from build123d import *

# Parameters (mm, degrees)
BOSS_EXTRUDE1_DEPTH = 4.5
SKETCH4_R           = 12.55
CUT_EXTRUDE1_DEPTH  = 2
CUT_EXTRUDE2_REACH  = 42.016
SKETCH5_R           = 2.1
SKETCH5_R_2         = 3.6
SKETCH8_W           = 3.5
SKETCH8_H           = 17
BOSS_EXTRUDE3_DEPTH = 20
FILLET3_R           = 10
FILLET4_R           = 10
SKETCH9_R           = 1.6
CUT_EXTRUDE3_DEPTH  = 68.190127898


with BuildPart() as part:
    # Sketch3 → Boss-Extrude1 (new body)
    with BuildSketch(Plane.XY):
        Polygon((-7.128665208, 13.142231947), (18.871334792, 13.142231947), (18.871334792, 2.142231947), (37.071334792, 2.142231947), (37.071334792, -14.857768053), (-25.328665208, -14.857768053), (-25.328665208, 2.142231947), (-7.128665208, 2.142231947), align=None)
    extrude(amount=BOSS_EXTRUDE1_DEPTH)

    # Sketch4 → Cut-Extrude1 (cut)
    with BuildSketch(Plane(origin=(0, 0, 0), x_dir=(-1, 0, 0), z_dir=(0, 0, -1))):
        with Locations((-5.871334792, 0.142231947)):
            Circle(SKETCH4_R)
    extrude(amount=-CUT_EXTRUDE1_DEPTH, mode=Mode.SUBTRACT)

    # Sketch5 → Cut-Extrude2 (cut, up to next)
    with BuildSketch(Plane(origin=(0, 0, 2), x_dir=(-1, 0, 0), z_dir=(0, 0, -1)), mode=Mode.PRIVATE) as cut_extrude2_sk1:
        with Locations((-14.621334792, 0.142231947)):
            Circle(SKETCH5_R)
    cut_extrude2_tool1 = extrude(cut_extrude2_sk1.sketch, amount=-CUT_EXTRUDE2_REACH, mode=Mode.PRIVATE) & part.part
    # Sketch5 → Cut-Extrude2 (cut, up to next)
    with BuildSketch(Plane(origin=(0, 0, 2), x_dir=(-1, 0, 0), z_dir=(0, 0, -1)), mode=Mode.PRIVATE) as cut_extrude2_sk2:
        with Locations(Location((2.878665208, 0.142231947, 0), (0, 0, 180))):
            Circle(SKETCH5_R)
    cut_extrude2_tool2 = extrude(cut_extrude2_sk2.sketch, amount=-CUT_EXTRUDE2_REACH, mode=Mode.PRIVATE) & part.part
    # Sketch5 → Cut-Extrude2 (cut, up to next)
    with BuildSketch(Plane(origin=(0, 0, 2), x_dir=(-1, 0, 0), z_dir=(0, 0, -1)), mode=Mode.PRIVATE) as cut_extrude2_sk3:
        with Locations((-5.871334792, 0.142231947)):
            Circle(SKETCH5_R_2)
    cut_extrude2_tool3 = extrude(cut_extrude2_sk3.sketch, amount=-CUT_EXTRUDE2_REACH, mode=Mode.PRIVATE) & part.part
    add(cut_extrude2_tool1.solids().sort_by_distance((14.621335, 0.142232, 2))[0], mode=Mode.SUBTRACT)
    add(cut_extrude2_tool2.solids().sort_by_distance((-2.878665, 0.142232, 2))[0], mode=Mode.SUBTRACT)
    add(cut_extrude2_tool3.solids().sort_by_distance((5.871335, 0.142232, 2))[0], mode=Mode.SUBTRACT)

    # Sketch8 → Boss-Extrude3 (add)
    with BuildSketch(Plane(origin=(0, 0, 0), x_dir=(-1, 0, 0), z_dir=(0, 0, -1))):
        with Locations((-35.321334792, -6.357768053)):
            Rectangle(SKETCH8_W, SKETCH8_H)
        with Locations((23.578665208, -6.357768053)):
            Rectangle(SKETCH8_W, SKETCH8_H)
    extrude(amount=BOSS_EXTRUDE3_DEPTH)

    # Fillet3
    fillet3_edges = [part.edges().sort_by_distance(p)[0] for p in [
        (-7.128665208, 2.142231947, 2.25),
        (18.871334792, 2.142231947, 2.25),
    ]]
    fillet(fillet3_edges, radius=FILLET3_R)

    # Fillet4
    fillet4_edges = [part.edges().sort_by_distance(p)[0] for p in [
        (-7.128665208, 13.142231947, 2.25),
        (18.871334792, 13.142231947, 2.25),
    ]]
    fillet(fillet4_edges, radius=FILLET4_R)

    # Sketch9 → Cut-Extrude3 (cut, through all)
    with BuildSketch(Plane(origin=(37.071334792, 0, 0), x_dir=(0, 0, -1), z_dir=(1, 0, 0))):
        with Locations((14, -3.357768053)):
            Circle(SKETCH9_R)
    extrude(amount=-CUT_EXTRUDE3_DEPTH, mode=Mode.SUBTRACT)


solid = part.part
Design review of the part built by this model. Coordinates are the model's own, in mm. A direction names the side the tool comes from. Round coordinates to 2 decimals unless told otherwise and drop trailing zeros. Loops run counter-clockwise (first coordinate to the right, second up) from the corner with the lowest first, then second, coordinate; pieces in that order, holes last. Notation, with made-up numbers: (73.25, -31.75) - (123.25, -31.75) arc R6 ccw to (123.25, -24.75) - close; hole circle Ø4 at (57.5, 34.25). An arc over 180 degrees is marked (long way). One line per question, with ' | ' between items.
1. We need section B-B, the plane z = -6. State the section outline as (x, y) points.
Results are:
outline: (-25.33, -14.86) - (-21.83, -14.86) - (-21.83, 2.14) - (-25.33, 2.14) - close; (33.57, -14.86) - (37.07, -14.86) - (37.07, 2.14) - (33.57, 2.14) - close
2. For faces 5 (the face through (9, -2, 2)), 6 (the face through (-21.829, -6, -10)), 7 (the face through (8.728, -2.048, 3.232)), list the 3-axis set-ups (+Z, -Z, +X, -X, +Y, -Y) from which the entire face can be reached by the end or side of a thin tool; tool diameter is ignored.
Results are:
face 5: -Z | face 6: -Z, +Y, -Y | face 7: +Z, -Z
3. Clearance check with flat-ended pins moving along their axes: P1, Ø1, axis at x = 6.5, y = 9.5, coming from the -Z side; P2, Ø12, axis at y = 7.5, z = -6.5, coming from the -X side; P3, Ø4, axis at x = 33, z = -3.5, coming from the +Y side. State where each tip first meets the part, or that it passes through.
Results are:
P1: stops at z = 2 | P2: stops at x = -25.33 | P3: stops at y = 2.14
4. We need section D-D, the plane y = 3. State the section outline as (x, z) points.
Results are:
outline: (-13.08, 0) - (-6.35, 0) - (-6.35, 2) - (3.68, 2) - (3.68, 4.5) - (-13.08, 4.5) - close; (8.06, 2) - (18.09, 2) - (18.09, 0) - (24.82, 0) - (24.82, 4.5) - (8.06, 4.5) - close
5. We need section A-A, the plane z = -14. State the section outline as (x, y) points.
Results are:
outline: (-25.33, -14.86) - (-21.83, -14.86) - (-21.83, -4.96) - (-25.33, -4.96) - close; (-25.33, -1.76) - (-21.83, -1.76) - (-21.83, 2.14) - (-25.33, 2.14) - close; (33.57, -14.86) - (37.07, -14.86) - (37.07, -4.96) - (33.57, -4.96) - close; (33.57, -1.76) - (37.07, -1.76) - (37.07, 2.14) - (33.57, 2.14) - close
6. Draft analysis for pull direction Y (two halves, no side actions). For faces 1 (the face through (8, -14.858, 1)), 2 (the face through (35, 2.142, -5)), 3 (the face through (16.72, 0.23, 3.23)), 4 (the face through (-6.1, 3.91, 0.99)), state which applies: released by +Y, released by -Y, zero draft, split by the parting line, or undercut.
Results are:
face 1: released by -Y | face 2: released by +Y | face 3: undercut | face 4: undercut
7. We need section C-C, the plane x = 4. State the section outline as (y, z) points.
Results are:
outline: (-14.86, 0) - (-12.27, 0) - (-12.27, 2) - (-2.93, 2) - (-2.93, 4.5) - (-14.86, 4.5) - close; (3.22, 2) - (12.55, 2) - (12.55, 0) - (13.14, 0) - (13.14, 4.5) - (3.22, 4.5) - close
8. For L1, parallel to X at y = -10.5, z = -0.75; L2, parallel to Y at x = -23.3, z = -14; L3, parallel to Z at x = -4, y = 5, list the stretches that pass through material, from the lowest coordinate up. Write a range as [from, to].
Results are:
L1: x = [-25.33, -21.83], [33.57, 37.07] | L2: y = [-14.86, -4.96], [-1.76, 2.14] | L3: z = [2, 4.5]
